Model file for the job. Use its own axes, mm. Coordinates: 2 decimals unless noted, no trailing zeros. Write each loop counter-clockwise with the first axis right and the second up, starting at its lowest first coordinate (ties: lowest second). Pieces come first, ordered by that corner, then holes. Notation, with made-up numbers: M 36,15 L 77,15 A21 cw 77,51 Z; hole C 4,76 d8. An arc over 180 degrees is marked long. Put each result on its own line as item: value. Start each with the question number.
Q1. Drill centre lines: line 1 along Y through (x, z) = (1.5, 432.5); line 2 along X through (y, z) = (17, 44.5); line 3 along X through (y, z) = (-2.5, 186). Where is each one in solid material? Low to high.
Q2. Drop flat-ended pins along their axis: pin 1 (12 mm diameter, centred on y = -13, z = 512.5, fed in from -X); pin 2 (1 mm diameter, centred on x = 8.5, z = 505.5, fed in from +Y); pin 3 (1.5 mm diameter, centred on x = 14.5, z = 224.5, fed in from -Y). Give the stop position or say it passes through.
Q3. Cut at C-C (y = 11.5). Write the cut outline in (x, z).
Q4. Cut at D-D (y = -11). Write the cut outline in (x, z).
Q5. Cut at B-B (z = 104). Write the cut outline in (x, y), then the cut area to 3 significant figures.
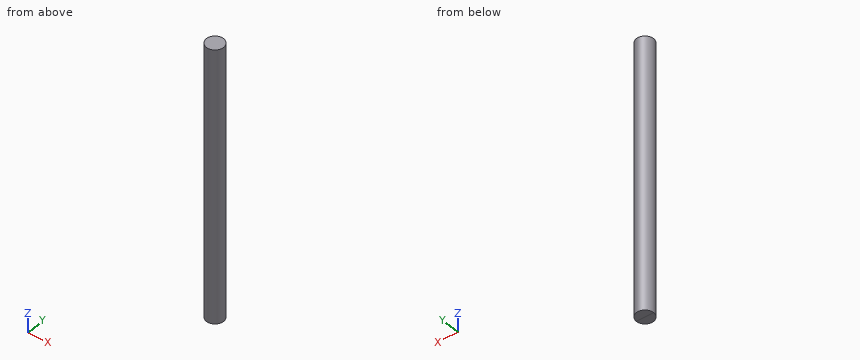
```python
from build123d import *

# Parameters (mm, degrees)
SKETCH1_R           = 19.05
BOSS_EXTRUDE2_DEPTH = 609.6
SKETCH2_W           = 38.1
SKETCH2_H           = 0.0005
CUT_EXTRUDE1_DEPTH  = 50.8
SKETCH5_W           = 38.1
SKETCH5_H           = 0.0005
CUT_EXTRUDE6_DEPTH  = 50.8


with BuildPart() as part:
    # Sketch1 → Boss-Extrude2 (new body)
    with BuildSketch(Plane.XY):
        Circle(SKETCH1_R)
    extrude(amount=BOSS_EXTRUDE2_DEPTH)

    # Sketch2 → Cut-Extrude1 (cut)
    with BuildSketch(Plane(origin=(0, 0, 0), x_dir=(-1, 0, 0), z_dir=(0, 0, -1))):
        with Locations((0, 0.00025)):
            Rectangle(SKETCH2_W, SKETCH2_H)
    extrude(amount=-CUT_EXTRUDE1_DEPTH, mode=Mode.SUBTRACT)

    # Sketch5 → Cut-Extrude6 (cut)
    with BuildSketch(Plane(origin=(0, 0, 0), x_dir=(-1, 0, 0), z_dir=(0, 0, -1))):
        with Locations((0, -0.00025)):
            Rectangle(SKETCH5_W, SKETCH5_H)
    extrude(amount=-CUT_EXTRUDE6_DEPTH, mode=Mode.SUBTRACT)


solid = part.part
```
Computed values:
1. line 1: -18.99 to 18.99
1. line 2: -8.6 to 8.6
1. line 3: -18.89 to 18.89
2. pin 1: x = -17.72
2. pin 2: y = 17.29
2. pin 3: y = -13.18
3. outline: M -15.19,0 L 15.19,0 L 15.19,609.6 L -15.19,609.6 Z
4. outline: M -15.55,0 L 15.55,0 L 15.55,609.6 L -15.55,609.6 Z
5. outline: C 0,0 d38.1
5. area: 1,140 mm2
